For this review, take the finished solid that the model builds, in its own axes (mm). Face numbers are marked on the shaded views. A direction names the side the tool comes from. Coordinates: 2 decimals unless noted, no trailing zeros. Write each loop counter-clockwise with the first axis right and the second up, starting at its lowest first coordinate (ties: lowest second). Pieces come first, ordered by that corner, then holes. Notation, with made-up numbers: (34, 27) - (52, 27) arc R14 ccw to (52, 34) - close; hole circle Ø11 at (38.25, -27). An arc over 180 degrees is marked (long way). Write each question's results on one line, items separated by ' | '.
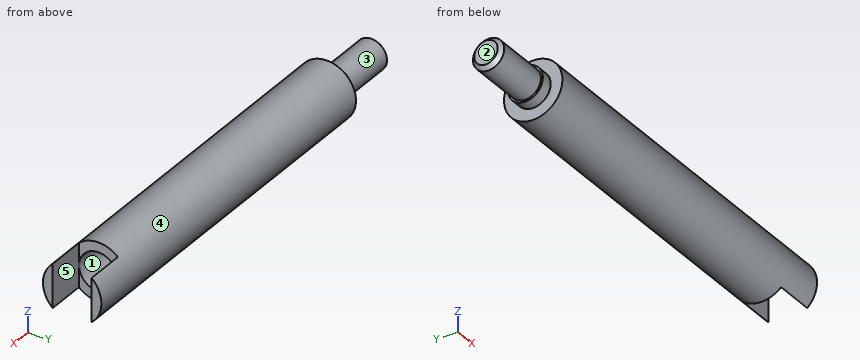
from build123d import *

# Parameters (mm, degrees)
CHAMFER_1_SIZE = 2
SKETCH1_W      = 30
SKETCH1_H      = 20
EXTRUDE1_DEPTH = 20
SKETCH2_R      = 10
EXTRUDE3_DEPTH = 160


with BuildPart() as part:
    # Эскиз1 → Повернуть1 (revolve)
    with BuildSketch(Plane.XY, mode=Mode.PRIVATE) as revolve_1_sk:
        Polygon((0, 0), (0, 8), (30, 8), (30, 9), (36, 9), (36, 15), (230, 15), (230, 0), align=None)
    revolve(revolve_1_sk.sketch.rotate(Axis((0, 0, 0), (-1, 0, 0)), 90), axis=Axis((0, 0, 0), (-1, 0, 0)))

    # Фаска1
    chamfer_1_edges = [part.edges().sort_by_distance(p)[0] for p in [
        (0, 0, 8),
    ]]
    chamfer(chamfer_1_edges, length=CHAMFER_1_SIZE)

    # Sketch1 → Extrude1 (cut)
    with BuildSketch(Plane(origin=(230, 0, 0), x_dir=(0, 0, -1), z_dir=(1, 0, 0))):
        Rectangle(SKETCH1_W, SKETCH1_H)
    extrude(amount=-EXTRUDE1_DEPTH, mode=Mode.SUBTRACT)

    # Sketch2 → Extrude3 (cut)
    with BuildSketch(Plane(origin=(210, 0, 0), x_dir=(0, 0, -1), z_dir=(1, 0, 0))):
        Circle(SKETCH2_R)
    extrude(amount=-EXTRUDE3_DEPTH, mode=Mode.SUBTRACT)


solid = part.part
Q1. For the marked faces 4 and 5, list the 3-axis set-ups (+Z, -Z, +X, -X, +Y, -Y) from which the entire face can be reached by the end or side of a thin tool; tool diameter is ignored.
Results found:
face 4: +X, -X | face 5: +Z, -Z, +X
Q2. Take a section at A-A on y = 0. State the section outline as (x, z) points, plus the area to 3 significant figures.
Results found:
outline: (0, -6) - (2, -8) - (30, -8) - (30, -9) - (36, -9) - (36, -15) - (210, -15) - (210, -10) - (50, -10) - (50, 10) - (210, 10) - (210, 15) - (36, 15) - (36, 9) - (30, 9) - (30, 8) - (2, 8) - (0, 6) - close | area: 2,600 mm2
Q3. Take a section at C-C on x = 118.5. State the section outline as (y, z) points, plus the area to 3 significant figures.
Results found:
outline: circle Ø30 at (0, 0); hole circle Ø20 at (0, 0) | area: 393 mm2
Q4. Take a section at D-D on x = 40.5. State the section outline as (y, z) points, plus the area to 3 significant figures.
Results found:
outline: circle Ø30 at (0, 0) | area: 707 mm2
Q5. Mouldability with a two-part tool opening along Z and no side actions: class the marked faces 1, 2 and 3 as pulls with the +Z half, pulls with the -Z half, needs draft (parallel to the pull), parting line crosses it, or undercut.
Results found:
face 1: undercut | face 2: needs draft | face 3: parting line crosses it
Q6. Wall thickness on line 1 along Y through (x, z) = (168.5, 0); line 2 along X through (y, z) = (8.25, -6); line 3 along Z through (x, y) = (52.5, 0.5): over which ranges is each line inside the solid? List them lowest first. Write a range as from..to.
Results found:
line 1: -15..-10, 10..15 | line 2: 36..210 | line 3: -14.99..-9.99, 9.99..14.99
Q7. For pin 1 (14.5 mm diameter, centred on y = -4, z = -2, fed in from -X); pin 2 (5 mm diameter, centred on y = -2.5, z = -4, fed in from +X); pin 3 (4 mm diameter, centred on x = 24.5, y = 1, fed in from +Z); pin 4 (5 mm diameter, centred on y = 6.5, z = 6.5, fed in from +X), all flat-tipped, find the tip position at first contact; note any pin that passes through.
Results found:
pin 1: x = 0 | pin 2: x = 50 | pin 3: z = 8 | pin 4: x = 210
Q8. Take a section at B-B on x = 215.5. State the section outline as (y, z) points, plus the area to 3 significant figures.
Results found:
outline: (-10, -11.18) - (-10, 11.18) arc R15 ccw to start; (10, -11.18) arc R15 ccw to (10, 11.18) - close | area: 155 mm2
